The model under review builds one solid part; all positions refer to its coordinate system, in mm. A direction names the side the tool comes from. Give positions to 0.01 mm unless a question says otherwise; leave off trailing zeros. Loops run counter-clockwise (first coordinate to the right, second up) from the corner with the lowest first, then second, coordinate; pieces in that order, holes last. Notation, with made-up numbers: M 15,-18 L 23,-18 A25 ccw 23,1 Z; hole C -22,39.5 d6. An arc over 180 degrees is marked long. Put each result on its own line as item: value. Start each with the question number.
from build123d import *

# Parameters (mm, degrees)
FILLET1_R = 3
FILLET2_R = 0.5


with BuildPart() as part:
    # base-sketch-2 → Revolve1 (revolve)
    with BuildSketch(Plane(origin=(0, 0, 0), x_dir=(1, 0, 0), z_dir=(0, 1, 0)), mode=Mode.PRIVATE) as revolve1_sk:
        Polygon((11, -26), (16.6, -18), (16.25, -18), (6, -18), (6, -26), align=None)
        Polygon((18.8956045, -0.741902481), (18, -0.741902481), (18, -3.95), (18, -16), (16.6, -18), (11, -26), (11, -31.630444462), (11.8956045, -31.630444462), (11.8956045, -26.630444462), (13, -26.630444462), (20, -16.630444462), (20, -4.741902481), (18.8956045, -4.741902481), align=None)
        Polygon((18, -16), (18, -3.95), (16.25, -16), (16.25, -18), (16.6, -18), align=None)
    revolve(revolve1_sk.sketch.rotate(Axis((0, 0, 0), (0, 0, 1)), 180), axis=Axis((0, 0, 0), (0, 0, 1)))

    # Fillet1
    fillet1_edges = [part.edges().sort_by_distance(p)[0] for p in [
        (20, 0, 16.630444462),
    ]]
    fillet(fillet1_edges, radius=FILLET1_R)

    # Fillet2
    fillet2_edges = [part.edges().sort_by_distance(p)[0] for p in [
        (13, 0, 26.630444462),
    ]]
    fillet(fillet2_edges, radius=FILLET2_R)


solid = part.part
(1) To check wall thickness, follow L1, parallel to Y at x = 0, z = 3.2; L2, parallel to Y at x = 0, z = 29.2; L3, parallel to Z at x = -6, y = -8. State the ranges of each line that lie inside material, in increasing order. Write a range as [from, to].
(2) We need section B-B, the plane z = 11.5. Write out the cut boundary in (x, y), plus the area to 3 significant figures.
(3) Draft analysis for pull direction Y (two halves, no side actions). For faces 4 (the cylindrical face through (19.98, -0.88, 10.14)), 5 (the flat face through (5, 5, 26)), 6 (the flat face through (-17, 7, 0.742)), state which applies: +Y half, -Y half, draft (parallel to the pull), parting line (faces both ways), or undercut.
(4) We need section A-A, the plane z = 23. Write out the cut boundary in (x, y).
(5) Insertion check: pin 1 (1.5 mm diameter, centred on x = -9.5, y = 13.5, fed in from +Z); pin 2 (5 mm diameter, centred on x = -9, z = 16, fed in from -Y); pin 3 (8 mm diameter, centred on x = -6, z = 18.5, fed in from -Y). Each pin has a flat end and moves straight along its axis. Give the tip position at first contact, or say it passes through.
(6) For faces 1 (the flat face through (12, 15, 4.742)), 2 (the flat face through (11, 3, 31.63)), 3 (the cylindrical face through (2.38, 10.74, 28.85)), list the 3-axis set-ups (+Z, -Z, +X, -X, +Y, -Y) from which the entire face can be reached by the end or side of a thin tool; tool diameter is ignored.
Check sheet entries:
1. L1: y = [-18.9, -18], [18, 18.9]
1. L2: y = [-11.9, -11], [11, 11.9]
1. L3: z = [18, 26]
2. outline: C 0,0 d40; hole C 0,0 d33.81
2. area: 359 mm²
3. face 4: parting line
3. face 5: undercut
3. face 6: draft
4. outline: C 0,0 d31.08; hole C 0,0 d12
5. pin 1: stops at z = 22.69
5. pin 2: stops at y = -18.91
5. pin 3: stops at y = -19.78
6. face 1: -Z
6. face 2: +Z, +X, -X, +Y, -Y
6. face 3: +Z
